```python
from build123d import *

# Parameters (mm, degrees)
BOSS_EXTRUDE3_DEPTH      = 15
BOSS_EXTRUDE3_DEPTH_BACK = 0.0001
CUT_EXTRUDE13_DEPTH      = 35.189972945
SKETCH31_W               = 5
SKETCH31_H               = 15
BOSS_EXTRUDE4_DEPTH      = 13.5
SKETCH32_W               = 5
SKETCH32_H               = 15.0001
BOSS_EXTRUDE5_DEPTH      = 13.5
BOSS_EXTRUDE6_REACH      = 44.929
SKETCH33_W               = 15
SKETCH33_H               = 8
CUT_EXTRUDE15_REACH      = 36.353
SKETCH34_R               = 1.75
SKETCH34_4_R             = 1.75
CUT_EXTRUDE16_DEPTH      = 15
FILLET1_R                = 5
FILLET2_R                = 5


with BuildPart() as part:
    # Sketch1 → Boss-Extrude3 (new, two sides: drawn at the far end of the back side and taken through both)
    with BuildSketch(Plane.XY.offset(-BOSS_EXTRUDE3_DEPTH_BACK)):
        with BuildLine():
            Line((-21.62638976, 2.067580939), (21.62638976, 2.067580939))
            ThreePointArc((21.62638976, 2.067580939), (0, -21.725), (-21.62638976, 2.067580939))
        make_face()
        with BuildLine():
            Line((18.013033205, -2.860307191), (-18.013033205, -2.860307191))
            ThreePointArc((-18.013033205, -2.860307191), (0, -18.238714935), (18.013033205, -2.860307191))
        make_face(mode=Mode.SUBTRACT)
    extrude(amount=BOSS_EXTRUDE3_DEPTH + BOSS_EXTRUDE3_DEPTH_BACK)

    # Sketch30 → Cut-Extrude13 (cut, through all)
    with BuildSketch(Plane.XY.offset(15)):
        with BuildLine():
            Line((-19.729884258, 0.067580939), (19.729884258, 0.067580939))
            ThreePointArc((19.729884258, 0.067580939), (0, -19.73), (-19.729884258, 0.067580939))
        make_face()
    extrude(amount=-CUT_EXTRUDE13_DEPTH, mode=Mode.SUBTRACT)

    # Sketch31 → Boss-Extrude4 (add)
    with BuildSketch(Plane(origin=(0, 2.067580939, 0), x_dir=(1, 0, 0), z_dir=(0, 1, 0))):
        with Locations((14.62638976, -7.4999)):
            Rectangle(SKETCH31_W, SKETCH31_H)
    extrude(amount=BOSS_EXTRUDE4_DEPTH)

    # Sketch32 → Boss-Extrude5 (add)
    with BuildSketch(Plane(origin=(0, 2.067580939, 0), x_dir=(1, 0, 0), z_dir=(0, 1, 0))):
        with Locations((-14.62638976, -7.49995)):
            Rectangle(SKETCH32_W, SKETCH32_H)
    extrude(amount=BOSS_EXTRUDE5_DEPTH)

    # Sketch33 → Boss-Extrude6 (add, up to next)
    with BuildSketch(Plane.ZY.offset(-12.12638976), mode=Mode.PRIVATE) as boss_extrude6_sk1:
        with Locations((7.4999, 11.567580939)):
            Rectangle(SKETCH33_W, SKETCH33_H)
    boss_extrude6_tool1 = extrude(boss_extrude6_sk1.sketch, amount=BOSS_EXTRUDE6_REACH, mode=Mode.PRIVATE) - part.part
    add(boss_extrude6_tool1.solids().sort_by_distance((12.12639, 11.567581, 7.4999))[0])

    # Sketch34 → Cut-Extrude15 (cut, up to next)
    with BuildSketch(Plane(origin=(0.255092403, 0, -0.0001), x_dir=(-1, 0, 0), z_dir=(0, 0, -1)), mode=Mode.PRIVATE) as cut_extrude15_sk1:
        with Locations((3.7956, 10.885680426)):
            Circle(SKETCH34_R)
    cut_extrude15_tool1 = extrude(cut_extrude15_sk1.sketch, amount=-CUT_EXTRUDE15_REACH, mode=Mode.PRIVATE) & part.part
    add(cut_extrude15_tool1.solids().sort_by_distance((-3.540508, 10.88568, -0.0001))[0], mode=Mode.SUBTRACT)

    # Sketch34<4> → Cut-Extrude16 (cut)
    with BuildSketch(Plane(origin=(0.255092403, 0, -0.0001), x_dir=(-1, 0, 0), z_dir=(0, 0, -1))):
        with Locations((-5.736564211, 10.885680426)):
            Circle(SKETCH34_4_R)
        with Locations((3.7956, 10.885680426)):
            Circle(SKETCH34_4_R)
    extrude(amount=-CUT_EXTRUDE16_DEPTH, mode=Mode.SUBTRACT)

    # Fillet1
    fillet1_edges = [part.edges().sort_by_distance(p)[0] for p in [
        (17.12638976, 15.567580939, 7.4999),
    ]]
    fillet(fillet1_edges, radius=FILLET1_R)

    # Fillet2
    fillet2_edges = [part.edges().sort_by_distance(p)[0] for p in [
        (-17.12638976, 15.567580939, 7.49995),
    ]]
    fillet(fillet2_edges, radius=FILLET2_R)


solid = part.part
```
Read the model definition and answer for the solid it produces. Units are mm, in the model's axes. A direction names the side the tool comes from. Coordinates: 2 decimals unless noted, no trailing zeros. Loops run counter-clockwise (first coordinate to the right, second up) from the corner with the lowest first, then second, coordinate; pieces in that order, holes last. Notation, with made-up numbers: (50, -12.75) -> (103, -12.75) arc R28 cw to (103, 12.25) -> close; hole circle Ø1 at (85, 88.5). An arc over 180 degrees is marked (long way). Return JSON: item names as keys, results as strings.
Item 1: Flat-ended cylindrical pins translate along their axes: P1, Ø7, axis at y = 9.5, z = 9.5, coming from the +X side; P2, Ø5, axis at y = 2, z = 3, coming from the -X side (3 decimals); P3, Ø4, axis at y = -9, z = 12, coming from the -X side; P4, Ø6, axis at y = -5, z = 3, coming from the -X side. Find the tip coordinate at first contact, or state that the pin passes through.
Answers:
{"P1": "stops at x = 17.13", "P2": "stops at x = -21.725", "P3": "stops at x = -20.57", "P4": "stops at x = -21.63"}
Item 2: Find section D-D (y = -1.5). Determine the outline of the cut face in (x, z), plus the area to 3 significant figures.
Answers:
{"outline": "(-21.67, 0) -> (-19.67, 0) -> (-19.67, 15) -> (-21.67, 15) -> close; (19.67, 0) -> (21.67, 0) -> (21.67, 15) -> (19.67, 15) -> close", "area": "60.0 mm2"}
Item 3: Find section B-B (x = 0). Determine the outline of the cut face in (y, z) (3 decimals).
Answers:
{"outline": "(-21.725, 0) -> (-19.73, 0) -> (-19.73, 15) -> (-21.725, 15) -> close; (0.068, 0) -> (2.068, 0) -> (2.068, 15) -> (0.068, 15) -> close; (7.568, 0) -> (15.568, 0) -> (15.568, 15) -> (7.568, 15) -> close"}
Item 4: Find the intervals of material crossed by probe 1 along X at (y, z) = (11, 11.25); probe 2 along Y at (x, z) = (-11.5, 7.75); probe 3 along Y at (x, z) = (9, 11), in increasing order.
Answers:
{"probe 1": "x = -17.11 to -5.29, -1.79 to 4.25, 7.74 to 17.11", "probe 2": "y = -18.43 to -16.03, 0.07 to 2.07, 7.57 to 15.57", "probe 3": "y = -19.77 to -17.56, 0.07 to 2.07, 7.57 to 15.57"}
Item 5: For faces 4 (the flat face through (-19, 2.068, 7)), 5 (the cylindrical face through (0.435, -19.725, 7.605)), 6 (the flat face through (17.126, 6, 8)), determine the directions among +Z, -Z, +X, -X, +Y, -Y from which every point of the face is accessible in a straight line to the end or side of a thin tool.
Answers:
{"face 4": "+Z, -Z, -X, +Y", "face 5": "+Z, -Z", "face 6": "+Z, -Z, +X, +Y"}
Item 6: For a pull along X with two mould halves and no side action, classify faces 1 (the flat face through (0, 1, 0)), 2 (the cylindrical face through (0.51, -21.72, 7.39)), 3 (the flat face through (0, 7.568, 7)) as +X half, -X half, draft (parallel to the pull), parting line (faces both ways), or undercut.
Answers:
{"face 1": "draft", "face 2": "parting line", "face 3": "undercut"}
Item 7: Find section A-A (y = 7). Determine the outline of the cut face in (x, z).
Answers:
{"outline": "(-17.13, 0) -> (-12.13, 0) -> (-12.13, 15) -> (-17.13, 15) -> close; (12.13, 0) -> (17.13, 0) -> (17.13, 15) -> (12.13, 15) -> close"}
Item 8: Find section C-C (z = 10.5). Count the separate pieces of the cut face and the enclosed holes in it, plus the area to 3 significant figures.
Answers:
{"separate pieces": "1", "enclosed holes": "4", "area": "516 mm2"}
